Autodesk Inventor part; units mm, degrees
ref_plane "YZ Plane" through (0, 0, 0) normal (1, 0, 0) x (0, 1, 0)
ref_plane "XZ Plane" through (0, 0, 0) normal (0, 1, 0) x (-1, 0, 0)
ref_plane "XY Plane" through (0, 0, 0) normal (0, 0, 1) x (1, 0, 0)
sketch "Sketch1" plane through (0, 0, 0) normal (0, 1, 0) x (-1, 0, 0)
  point P0 (0, 0)
sketch "Sketch2" plane through (0, 0, 0) normal (0, 1, 0) x (-1, 0, 0)
  circle A0 centre (0, 0) radius 17.78
  circle A1 centre (0, 0) radius 9.525
  dimension "d0" = 35.56
  dimension "d1" = 19.05
extrude "Extrusion1" add sketch "Sketch2" along normal blind 50.8
chamfer "Chamfer1" distance 0.3175 angle 45 2 edges at (9.525, 50.8, 0) (17.78, 0, 0)
sketch "Sketch3" plane through (0, 50.8, 0) normal (0, 1, 0) x (1, 0, 0)
  line L0 (-20.433, 19.5533) -> (20.433, 19.5533)
  line L1 (20.433, 19.5533) -> (20.433, -19.5533)
  line L2 (20.433, -19.5533) -> (-20.433, -19.5533)
  line L3 (-20.433, -19.5533) -> (-20.433, 19.5533)
  line L4 (-20.433, 19.5533) -> (20.433, -19.5533) construction
  line L5 (20.433, 19.5533) -> (-20.433, -19.5533) construction
  line L6 (-14.9596, 14.3155) -> (14.9596, 14.3155)
  line L7 (14.9596, 14.3155) -> (14.9596, -14.3155)
  line L8 (14.9596, -14.3155) -> (-14.9596, -14.3155)
  line L9 (-14.9596, -14.3155) -> (-14.9596, 14.3155)
  line L10 (-14.9596, 14.3155) -> (14.9596, -14.3155) construction
  line L11 (14.9596, 14.3155) -> (-14.9596, -14.3155) construction
  line L12 (-9.4862, -9.0778) -> (-20.433, -9.0778)
  line L13 (-20.433, -9.0778) -> (-20.433, -19.5533)
  line L14 (-20.433, -19.5533) -> (-9.4862, -19.5533)
  line L15 (-9.4862, -19.5533) -> (-9.4862, -9.0778)
  line L16 (-9.4862, -9.0778) -> (-20.433, -19.5533) construction
  line L17 (-20.433, -9.0778) -> (-9.4862, -19.5533) construction
  circle A0 centre (0, 0) radius 13.1299
extrude "Extrusion2" add sketch "Sketch3" along normal blind 2.54 contours L0 L1 L2 L15 L8 L7 L6 L9 L12 L3 | L9 L6 L7 L8 L15 L12
properties part number "Wheel Washer"
CAD build for the part. Positions are in the model's coordinates, mm. A direction names the side the tool comes from. Give positions to 0.01 mm unless a question says otherwise; leave off trailing zeros. Order: outer loops, then holes, each group sorted by start corner. A loop starts at its lowest first (then second) coordinate and runs counter-clockwise, first axis right, second up.
(1) Saw through at A-A, the plane x = 0. Give the cut face in (y, z) (1 decimal).
(2) Drill centre lines: L1, parallel to Z at x = 0, y = 51; L2, parallel to Z at x = 0, y = 38 (3 decimals); L3, parallel to X at y = 52.3, z = 0. Where is each one in solid material? Low to high.
(3) Saw through at B-B, the plane y = 41. Give the cut face in (x, z) (3 decimals).
(4) Mould opens along Z. For faces 1 (the flat face through (-9.486, 52, 14)), 2 (the flat face through (0, 52, -19.553)), 3 (the flat face through (2, 50.8, -10)) say: released by +Z, released by -Z, zero draft, split by the parting line, or undercut.
(5) Tool access for faces 4 (the flat face through (-0.3, 53.34, -13.3)), 5 (the flat face through (18, 50.8, 0)), 6 (the flat face through (-15, 52, 9.078)): list every direction of +Z, -Z, +X, -X, +Y, -Y with a clear straight run to the whole face (end or side of a thin tool).
(6) Flat gauge pins, fed straight in: pin 1 (2 mm diameter, centred on x = 15.5, y = 40.5, fed in from +Z); pin 2 (10 mm diameter, centred on y = 32.5, z = 13, fed in from +X); pin 3 (1.7 mm diameter, centred on x = -12.5, z = 11, fed in from +Y); pin 4 (15 mm diameter, centred on x = 0, z = 0, fed in from +Y). Where does each tip first touch, or does it go through?
Results found:
1. outline: (0, -17.5) - (0.3, -17.8) - (50.8, -17.8) - (50.8, -19.6) - (53.3, -19.6) - (53.3, -13.1) - (50.8, -13.1) - (50.8, -9.8) - (50.5, -9.5) - (0, -9.5) - close; (0, 9.5) - (50.5, 9.5) - (50.8, 9.8) - (50.8, 13.1) - (53.3, 13.1) - (53.3, 19.6) - (50.8, 19.6) - (50.8, 17.8) - (0.3, 17.8) - (0, 17.5) - close
2. L1: z = -19.55 to -13.13, 13.13 to 19.55
2. L2: z = -17.78 to -9.525, 9.525 to 17.78
2. L3: x = -20.43 to -13.13, 13.13 to 20.43
3. outline: circle Ø35.56 at (0, 0); hole circle Ø19.05 at (0, 0)
4. face 1: zero draft
4. face 2: released by -Z
4. face 3: undercut
5. face 4: +Z, -Z, +X, -X, +Y
5. face 5: -Y
5. face 6: +Z, -X, +Y
6. pin 1: stops at z = 10.29
6. pin 2: stops at x = 15.88
6. pin 3: stops at y = 50.8
6. pin 4: passes through
